Read the model definition and answer for the solid it produces. Units are mm, in the model's axes. Face numbers are marked on the shaded views. Round coordinates to 2 decimals unless told otherwise and drop trailing zeros. Write each loop counter-clockwise with the first axis right and the second up, starting at its lowest first coordinate (ties: lowest second). Pieces come first, ordered by that corner, then holes. Notation, with made-up numbers: (51.25, 46.5) - (95.25, 46.5) arc R16 cw to (95.25, 77.5) - close; hole circle Ø4 at (21, 42.5). An arc over 180 degrees is marked (long way). Answer as CSV lines item,"result". Start each with the question number.
1) Consider line 1 along Z through (x, y) = (8.5, 2.2); line 2 along X through (y, z) = (1.75, 9); line 3 along Z through (x, y) = (-0.25, 2.1). Determine where each line is inside the solid, lowest interval first.
2) Find section B-B on z = 9. Determine the outline of the cut face in (x, y).
3) For a pull along Z with two mould halves and no side action, classify the marked faces 1, 2 and 3 as +Z half, -Z half, draft (parallel to the pull), parting line (faces both ways), or undercut.
4) Find section C-C on y = 0.3. Determine the outline of the cut face in (x, z), then the cut area to 3 significant figures.
5) Find section A-A on x = 8.5. Determine the outline of the cut face in (y, z), then the cut area to 3 significant figures.
6) Each of these flat-tipped pins is pushed along its axis until it touches: pin 1 (1.4 mm diameter, centred on x = -1, y = 2, fed in from +Z); pin 2 (0.5 mm diameter, centred on y = 2, z = 12, fed in from -X). Where does it stop, or does it pass through?
Autodesk Inventor part; units mm, degrees
ref_plane "YZ Plane" through (0, 0, 0) normal (1, 0, 0) x (0, 1, 0)
ref_plane "XZ Plane" through (0, 0, 0) normal (0, 1, 0) x (-1, 0, 0)
ref_plane "XY Plane" through (0, 0, 0) normal (0, 0, 1) x (1, 0, 0)
ref_plane "Work Plane1" through (0, 0, 5) normal (0, 0, 1) x (1, 0, 0)
sketch "Sketch1" plane through (0, 0, 5) normal (0, 0, 1) x (1, 0, 0)
  line L0 (0, 0) -> (20, 0)
  line L1 (20, 0) -> (20, 2.9)
  line L2 (20, 2.9) -> (0, 2.9)
  line L3 (0, 2.9) -> (0, 0)
  dimension "d2" = 20
  dimension "d1" = 2.9
extrude "Extrusion1" add sketch "Sketch1" along normal blind 8
sketch "Sketch2" plane through (0, 0, 5) normal (-1, 0, 0) x (0, 0, 1)
  line L0 (0, 0) -> (0, 2.9)
  line L1 (0, 0) -> (8, 0)
  line L2 (0, 0) -> (6.2, 0)
  line L3 (6.2, 0) -> (6.2, 2.9)
  line L4 (6.2, 2.9) -> (0, 2.9)
  line L5 (0, 2.9) -> (0, 0)
  point P0 (-13, 0)
  dimension "d6" = 6.2
extrude "Extrusion2" add sketch "Sketch2" along normal blind 3
sketch "Sketch3" plane through (20, 2.9, 5) normal (0, 1, 0) x (0, 0, 1)
  line L0 (0, 0) -> (0, -23)
  line L1 (8, -20) -> (8, 0)
  line L2 (0, -20) -> (8, -20)
  line L3 (4, -20) -> (4, -11.5)
  circle A0 centre (4, -11.5) radius 2
  point P0 (-13, -20)
  dimension "d11" = 8.5
  dimension "d10" = 4
extrude "Extrusion3" cut sketch "Sketch3" against normal through all
properties part number "Cap Pulley Support V2 Pt2" material "Thermoplastic Resin"
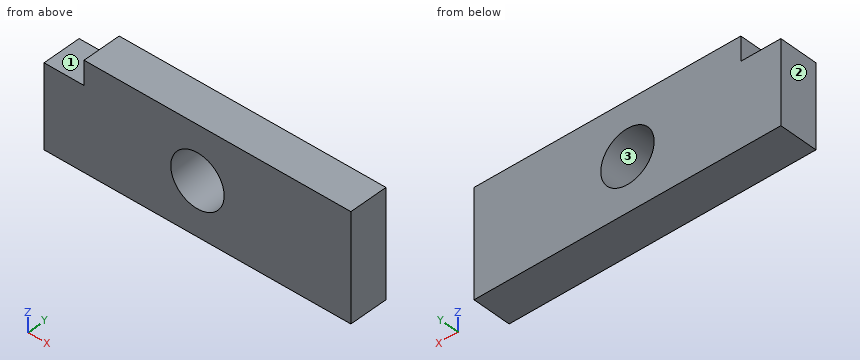
Check values:
1,line 1,"z = 5 to 7, 11 to 13"
1,line 2,"x = -3 to 6.5, 10.5 to 20"
1,line 3,"z = 5 to 11.2"
2,outline,"(-3, 0) - (6.5, 0) - (6.5, 2.9) - (-3, 2.9) - close; (10.5, 0) - (20, 0) - (20, 2.9) - (10.5, 2.9) - close"
3,face 1,"+Z half"
3,face 2,"draft"
3,face 3,"undercut"
4,outline,"(-3, 5) - (20, 5) - (20, 13) - (0, 13) - (0, 11.2) - (-3, 11.2) - close; hole circle Ø4 at (8.5, 9)"
4,area,"166 mm^2"
5,outline,"(0, 5) - (2.9, 5) - (2.9, 7) - (0, 7) - close; (0, 11) - (2.9, 11) - (2.9, 13) - (0, 13) - close"
5,area,"11.6 mm^2"
6,pin 1,"stops at z = 11.2"
6,pin 2,"stops at x = 0"
